Job drawing, mm, ordinate dimensions from the low corner. One solid piece. Coordinates: 2 decimals unless noted, no trailing zeros. Loops run counter-clockwise (first coordinate to the right, second up) from the corner with the lowest first, then second, coordinate; pieces in that order, holes last. Notation, with made-up numbers: (11, -4.5) - (30, -4.5) arc R10 ccw to (30, 14.5) - close; hole circle Ø2 at (5, 12.5). An arc over 180 degrees is marked (long way). Use a Markdown table: item, result. Add a question column.
1) Band-saw the part on C-C (z = 7). Give the number of separate pieces and of enclosed holes in the cut face, plus the area to 3 significant figures.
2) Band-saw the part on D-D (z = 1.25). Give the cut face in (x, y).
3) Probe probe 1 along Y at (x, z) = (50, 6); probe 2 along Y at (x, z) = (72, 9) (1 decimal); probe 3 along Z at (x, y) = (47.5, 86). List the from-to ranges inside material, lowest first. Write a range as [from, to].
4) Band-saw the part on A-A (x = 50). Give the cut face in (y, z).
5) Drop flat-ended pins along their axis: P1, Ø1, axis at y = 66, z = 8.5, coming from the -X side; P2, Ø5, axis at x = 33.5, z = 8, coming from the -Y side; P3, Ø3, axis at x = 50, y = 89.5, coming from the +Z side. Give the stop position or say it passes through.
6) Band-saw the part on B-B (y = 38.5). Give the cut face in (x, z).
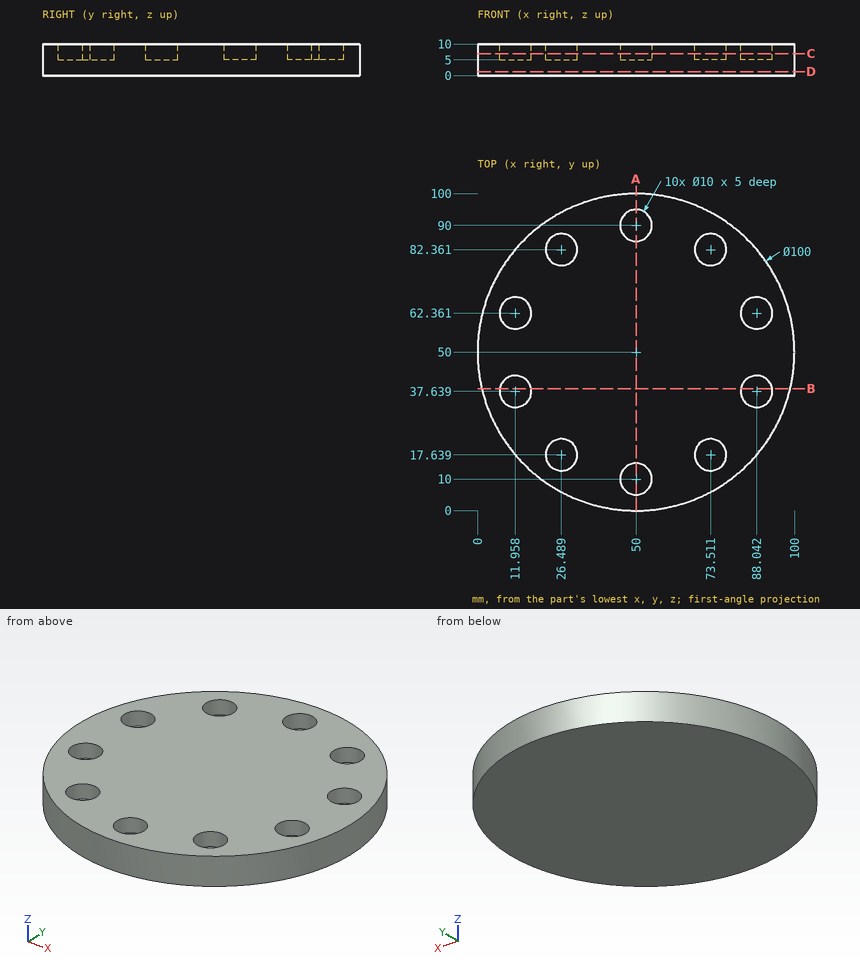
Answer block:
| question | item | result |
|---|---|---|
| 1 | separate pieces | 1 |
| 1 | enclosed holes | 10 |
| 1 | area | 7,070 mm2 |
| 2 | outline | circle Ø100 at (50, 50) |
| 3 | probe 1 | [0, 5], [15, 85], [95, 100] |
| 3 | probe 2 | [5.1, 12.9], [22.4, 77.6], [87.1, 94.9] |
| 3 | probe 3 | [0, 5] |
| 4 | outline | (0, 0) - (100, 0) - (100, 10) - (95, 10) - (95, 5) - (85, 5) - (85, 10) - (15, 10) - (15, 5) - (5, 5) - (5, 10) - (0, 10) - close |
| 5 | P1 | x = 2.46 |
| 5 | P2 | y = 2 |
| 5 | P3 | z = 5 |
| 6 | outline | (1.34, 0) - (98.66, 0) - (98.66, 10) - (92.97, 10) - (92.97, 5) - (83.12, 5) - (83.12, 10) - (16.88, 10) - (16.88, 5) - (7.03, 5) - (7.03, 10) - (1.34, 10) - close |
